The listing builds one solid part. Answer for the finished solid, in the listing's coordinates (mm). A direction names the side the tool comes from. Round coordinates to 2 decimals unless told otherwise and drop trailing zeros. Write each loop counter-clockwise with the first axis right and the second up, starting at its lowest first coordinate (ties: lowest second). Pieces come first, ordered by that corner, then holes.
(1) The mould has two halves that part along X. Classify faces 6 (the face through (29.055, -8.628, -141.812)), 7 (the face through (3, 3, -35)), 8 (the face through (33.31, -8.63, -33.96)): +X half, -X half, draft (parallel to the pull), parting line (faces both ways), or undercut.
(2) A cutting plane is placed at C-C, the plane x = 21.5. Give the vertices of the cut face in (y, z).
(3) A cutting plane is placed at A-A, the plane y = -15.5. Give the vertices of the cut face in (x, z), and give its area (3 significant figures).
(4) A cutting plane is placed at B-B, the plane z = -87.5. Give the vertices of the cut face in (x, y), and give its area (3 significant figures).
(5) Each of these flat-tipped pins is pushed along its axis until it touches: pin 1 Ø5.5 at (y, z) = (2.5, -2.5) entering from +X; pin 2 Ø4.5 at (x, y) = (15.5, 3) entering from -Z; pin 3 Ø1.5 at (x, y) = (29.5, -1.5) entering from +Z; pin 4 Ø2 at (x, y) = (25, -8) entering from +Z. Where does it stop, or does it pass through?
(6) Find the intervals of material crossed by probe 1 along Z at (x, y) = (57, 4); probe 2 along Y at (x, z) = (83, -8); probe 3 along Z at (x, y) = (151.5, 2.75), in increasing order.
(7) For faces 1 (the face through (62.81, 2.71, -67.05)), 2 (the face through (35, 3, -173)), 3 (the face through (140, 3, -172)), 4 (the face through (172, 3, -35)), 5 (the face through (141.042, -8.628, -29.014)), determine the directions among +Z, -Z, +X, -X, +Y, -Y from which every point of the face is accessible in a straight line to the end or side of a thin tool.
from build123d import *

# Parameters (mm, degrees)
SKETCH_1_R      = 15
EXTRUDE_2_DEPTH = 5.5
EXTRUDE_3_DEPTH = 23


with BuildPart() as part:
    # Эскиз1 → Бобышка-Вытянуть2 (new body)
    with BuildSketch(Plane(origin=(0, 0, 0), x_dir=(1, 0, 0), z_dir=(0, 1, 0))):
        Polygon((170, 140), (170, 170), (140, 170), (140, 175), (105, 175), (105, 170), (70, 170), (70, 175), (35, 175), (35, 170), (0, 170), (0, 140), (5, 140), (5, 105), (0, 105), (0, 70), (5, 70), (5, 35), (0, 35), (0, 0), (35, 0), (35, 5), (70, 5), (70, 0), (105, 0), (105, 5), (140, 5), (140, 0), (170, 0), (170, 35), (175, 35), (175, 70), (170, 70), (170, 105), (175, 105), (175, 140), align=None)
        Polygon((19.339817755, 14.98716546), (30.853332638, 26.500680342), (42.36684752, 14.98716546), align=None, mode=Mode.SUBTRACT)
        Polygon((26.610691951, 30.743321029), (15.097177068, 19.229806147), (15.097177068, 42.256835911), align=None, mode=Mode.SUBTRACT)
        with BuildLine():
            ThreePointArc((54.899758827, 50.65711814), (87.41386875, 38.50044692), (119.822950774, 50.934408539))
            Line((119.822950774, 50.934408539), (134.689086203, 36.06827311))
            ThreePointArc((134.689086203, 36.06827311), (87.41366824, 17.500312244), (40.028175023, 35.785534336))
            Line((40.028175023, 35.785534336), (54.899758827, 50.65711814))
        make_face(mode=Mode.SUBTRACT)
        with BuildLine():
            Line((35.772862168, 134.984497145), (50.638997596, 120.118361717))
            ThreePointArc((50.638997596, 120.118361717), (38.204589058, 87.5), (50.638997596, 54.881638283))
            Line((50.638997596, 54.881638283), (35.772862168, 40.015502855))
            ThreePointArc((35.772862168, 40.015502855), (17.204589058, 87.5), (35.772862168, 134.984497145))
        make_face(mode=Mode.SUBTRACT)
        with BuildLine():
            ThreePointArc((74.798754674, 70.556113987), (87.415641051, 66.501060573), (99.948475479, 70.808883834))
            Line((99.948475479, 70.808883834), (115.572444887, 55.184914426))
            ThreePointArc((115.572444887, 55.184914426), (87.413986392, 44.500509855), (59.152804826, 54.910164139))
            Line((59.152804826, 54.910164139), (74.798754674, 70.556113987))
        make_face(mode=Mode.SUBTRACT)
        Polygon((155.770193853, 14.98716546), (132.743164089, 14.98716546), (144.256678971, 26.500680342), align=None, mode=Mode.SUBTRACT)
        Polygon((160.01283454, 19.229806147), (148.499319658, 30.743321029), (160.01283454, 42.256835911), align=None, mode=Mode.SUBTRACT)
        with BuildLine():
            Line((54.889503484, 115.867855829), (70.513472891, 100.243886422))
            ThreePointArc((70.513472891, 100.243886422), (66.204589058, 87.5), (70.513472891, 74.756113578))
            Line((70.513472891, 74.756113578), (54.889503484, 59.132144171))
            ThreePointArc((54.889503484, 59.132144171), (44.204589058, 87.5), (54.889503484, 115.867855829))
        make_face(mode=Mode.SUBTRACT)
        with BuildLine():
            Line((115.572444887, 119.815085574), (99.948475479, 104.191116166))
            ThreePointArc((99.948475479, 104.191116166), (87.415641051, 108.498939427), (74.798754674, 104.443886013))
            Line((74.798754674, 104.443886013), (59.152804826, 120.089835861))
            ThreePointArc((59.152804826, 120.089835861), (87.413986392, 130.499490145), (115.572444887, 119.815085574))
        make_face(mode=Mode.SUBTRACT)
        Polygon((15.097177068, 132.743164089), (15.097177068, 155.770193853), (26.610691951, 144.256678971), align=None, mode=Mode.SUBTRACT)
        Polygon((19.339817755, 160.01283454), (42.36684752, 160.01283454), (30.853332638, 148.499319658), align=None, mode=Mode.SUBTRACT)
        with BuildLine():
            Line((134.689086203, 138.93172689), (119.822950774, 124.065591461))
            ThreePointArc((119.822950774, 124.065591461), (87.41386875, 136.49955308), (54.899758827, 124.34288186))
            Line((54.899758827, 124.34288186), (40.028175023, 139.214465664))
            ThreePointArc((40.028175023, 139.214465664), (87.41366824, 157.499687756), (134.689086203, 138.93172689))
        make_face(mode=Mode.SUBTRACT)
        with Locations((87.204589058, 87.5)):
            Circle(SKETCH_1_R, mode=Mode.SUBTRACT)
        with BuildLine():
            ThreePointArc((104.148475071, 75.094165616), (108.204589058, 87.5), (104.148475071, 99.905834384))
            Line((104.148475071, 99.905834384), (119.794424918, 115.551784231))
            ThreePointArc((119.794424918, 115.551784231), (130.204589058, 87.5), (119.794424918, 59.448215769))
            Line((119.794424918, 59.448215769), (104.148475071, 75.094165616))
        make_face(mode=Mode.SUBTRACT)
        with BuildLine():
            ThreePointArc((124.047470918, 55.195169769), (136.204589058, 87.5), (124.047470918, 119.804830231))
            Line((124.047470918, 119.804830231), (138.919054721, 134.676414034))
            ThreePointArc((138.919054721, 134.676414034), (157.204589058, 87.5), (138.919054721, 40.323585966))
            Line((138.919054721, 40.323585966), (124.047470918, 55.195169769))
        make_face(mode=Mode.SUBTRACT)
        Polygon((160.01283454, 132.743164089), (148.499319658, 144.256678971), (160.01283454, 155.770193853), align=None, mode=Mode.SUBTRACT)
        Polygon((132.743164089, 160.01283454), (155.770193853, 160.01283454), (144.256678971, 148.499319658), align=None, mode=Mode.SUBTRACT)
    extrude(amount=EXTRUDE_2_DEPTH)

    # Эскиз2 → Бобышка-Вытянуть3 (add)
    with BuildSketch(Plane(origin=(0, 5.5, 0), x_dir=(1, 0, 0), z_dir=(0, 1, 0))):
        Polygon((30.853332638, 148.499319658), (26.610691951, 144.256678971), (31.568480277, 139.298890644), (35.811120964, 143.541531331), align=None)
        Polygon((148.203908716, 143.85125642), (143.961268028, 148.093897107), (139.003479702, 143.136108781), (143.246120389, 138.893468093), align=None)
        Polygon((143.555845478, 26.500680342), (147.798486165, 30.743321029), (142.840697838, 35.701109356), (138.598057151, 31.458468669), align=None)
        Polygon((26.2052694, 31.14874358), (30.447910087, 26.906102893), (35.405698413, 31.863891219), (31.163057726, 36.106531907), align=None)
    extrude(amount=-EXTRUDE_3_DEPTH)


solid = part.part
Solutions:
1. face 6: -X half
1. face 7: draft
1. face 8: undercut
2. outline: (0, -170) - (5.5, -170) - (5.5, -160.01) - (0, -160.01) - close; (0, -157.85) - (5.5, -157.85) - (5.5, -149.37) - (0, -149.37) - close; (0, -139.15) - (5.5, -139.15) - (5.5, -111.64) - (0, -111.64) - close; (0, -63.36) - (5.5, -63.36) - (5.5, -35.85) - (0, -35.85) - close; (0, -25.63) - (5.5, -25.63) - (5.5, -17.15) - (0, -17.15) - close; (0, -14.99) - (5.5, -14.99) - (5.5, 0) - (0, 0) - close
3. outline: (26.21, -31.15) - (31.16, -36.11) - (35.41, -31.86) - (30.45, -26.91) - close; (26.61, -144.26) - (30.85, -148.5) - (35.81, -143.54) - (31.57, -139.3) - close; (138.6, -31.46) - (142.84, -35.7) - (147.8, -30.74) - (143.56, -26.5) - close; (139, -143.14) - (143.96, -148.09) - (148.2, -143.85) - (143.25, -138.89) - close
3. area: 168 mm2
4. outline: (0, 0) - (17.2, 0) - (17.2, 5.5) - (0, 5.5) - close; (38.2, 0) - (44.2, 0) - (44.2, 5.5) - (38.2, 5.5) - close; (66.2, 0) - (72.2, 0) - (72.2, 5.5) - (66.2, 5.5) - close; (102.2, 0) - (108.2, 0) - (108.2, 5.5) - (102.2, 5.5) - close; (130.2, 0) - (136.2, 0) - (136.2, 5.5) - (130.2, 5.5) - close; (157.2, 0) - (170, 0) - (170, 5.5) - (157.2, 5.5) - close
4. area: 297 mm2
5. pin 1: stops at x = 170
5. pin 2: stops at z = -170
5. pin 3: stops at z = -27.1
5. pin 4: passes through
6. probe 1: z = -175 to -150.65, -126.08 to -113.76, -61.24 to -48.92, -24.35 to -5
6. probe 2: y = 0 to 5.5
6. probe 3: z = -170 to -160.01, -155.74 to -147.26, -141.26 to -115.18, -59.82 to -33.74, -27.74 to -19.26, -14.99 to 0
7. face 1: +Y, -Y
7. face 2: -Z, -X, +Y, -Y
7. face 3: -Z, +X, +Y, -Y
7. face 4: +Z, +X, +Y, -Y
7. face 5: +Z, -Y
